from build123d import *

# Parameters (mm, degrees)
F1_DEPTH  = 35
F0_W      = 1.8
F0_H      = 39.6
F2_DEPTH  = 36
F0_W_2    = 30
F0_H_2    = 6.9
F3_DEPTH  = 1.8
F4_W      = 47.8
F4_H      = 28
F5_DEPTH  = 18
F4_W_2    = 50.8
F4_H_2    = 31.6
F6_DEPTH  = 1
F7_W      = 43.3
F7_H      = 39.6
F7_W_2    = 30
F7_H_2    = 48.3
F8_DEPTH  = 1.2
F0_W_3    = 6
F9_DEPTH  = 2
F10_R     = 1.6
F11_DEPTH = 2
F12_R     = 5.5
F13_DEPTH = 5
F10_R_2   = 4.5
F14_DEPTH = 2


with BuildPart() as f1:
    # F0 (on Top) → F1 (new body)
    with BuildSketch(Plane.XY):
        Polygon((-38.45, 21.6), (-38.45, 19.8), (-36.65, 19.8), (6.65, 19.8), (8.45, 19.8), (8.45, 21.6), (6.65, 21.6), align=None)
        Polygon((8.45, 21.6), (8.45, 19.8), (32.45, 19.8), (38.45, 19.8), (38.45, 21.6), align=None)
        Polygon((-36.65, -19.8), (-38.45, -19.8), (-38.45, -23.7), (40.25, -23.7), (40.25, 21.6), (38.45, 21.6), (38.45, 19.8), (38.45, -19.8), (32.45, -19.8), (12.45, -19.8), (12.45, -22.5), (-7.55, -22.5), (-7.55, -19.8), align=None)
    extrude(amount=F1_DEPTH)

    # F0 (on Top) → F2 (join)
    with BuildSketch(Plane.XY):
        with Locations((-37.55, 0)):
            Rectangle(F0_W, F0_H)
        Polygon((-38.45, 21.6), (-38.45, 19.8), (-36.65, 19.8), (6.65, 19.8), (8.45, 19.8), (8.45, 21.6), (6.65, 21.6), align=None)
        Polygon((6.65, 30.3), (6.65, 21.6), (8.45, 21.6), (8.45, 28.5), (38.45, 28.5), (38.45, 21.6), (40.25, 21.6), (40.25, 30.3), align=None)
        Polygon((-36.65, -19.8), (-38.45, -19.8), (-38.45, -23.7), (40.25, -23.7), (40.25, 21.6), (38.45, 21.6), (38.45, 19.8), (38.45, -19.8), (32.45, -19.8), (12.45, -19.8), (12.45, -22.5), (-7.55, -22.5), (-7.55, -19.8), align=None)
        Polygon((8.45, -19.8), (6.65, -19.8), (-7.55, -19.8), (-7.55, -22.5), (12.45, -22.5), (12.45, -19.8), align=None)
        with Locations((7.55, 0)):
            Rectangle(F0_W, F0_H)
    extrude(amount=-F2_DEPTH)

    # F0 (on Top) → F3 (join)
    with BuildSketch(Plane.XY):
        with Locations((23.45, 25.05)):
            Rectangle(F0_W_2, F0_H_2)
        Polygon((8.45, 21.6), (8.45, 19.8), (32.45, 19.8), (38.45, 19.8), (38.45, 21.6), align=None)
    extrude(amount=-F3_DEPTH)

    # F4 (on face) → F5 (cut)
    with BuildSketch(Plane.YZ.offset(40.25)):
        with Locations((3.3, -18)):
            Rectangle(F4_W, F4_H)
    extrude(amount=-F5_DEPTH, mode=Mode.SUBTRACT)

    # F4 (on face) → F6 (cut)
    with BuildSketch(Plane.YZ.offset(40.25)):
        with Locations((3.3, -18)):
            Rectangle(F4_W_2, F4_H_2)
        with Locations((3.3, -18)):
            Rectangle(F4_W, F4_H, mode=Mode.SUBTRACT)
    extrude(amount=-F6_DEPTH, mode=Mode.SUBTRACT)

    # F7 (on face) → F8 (join)
    with BuildSketch(Plane(origin=(0, 0, -36), x_dir=(1, 0, 0), z_dir=(0, 0, -1))):
        with Locations((-15, 0)):
            Rectangle(F7_W, F7_H)
        with Locations((23.45, -4.35)):
            Rectangle(F7_W_2, F7_H_2)
    extrude(amount=-F8_DEPTH)

    # F0 (on Top) → F9 (join)
    with BuildSketch(Plane.XY):
        with Locations((35.45, 0)):
            Rectangle(F0_W_3, F0_H)
    extrude(amount=-F9_DEPTH)

    # F10 (on face) → F11 (cut)
    with BuildSketch(Plane(origin=(0, 21.6, 0), x_dir=(-1, 0, 0), z_dir=(0, 1, 0))):
        with Locations((-35.25, 12.1)):
            Circle(F10_R)
    extrude(amount=-F11_DEPTH, mode=Mode.SUBTRACT)

    # F12 (on face) → F13 (cut)
    with BuildSketch(Plane(origin=(-38.45, 0, 0), x_dir=(0, -1, 0), z_dir=(-1, 0, 0))):
        with Locations((-3, -9)):
            Circle(F12_R)
        with Locations((16.8, -9)):
            Circle(F12_R)
        with Locations((6.9, -28.8)):
            Circle(F12_R)
    extrude(amount=-F13_DEPTH, mode=Mode.SUBTRACT)

    # F10 (on face) → F14 (cut)
    with BuildSketch(Plane(origin=(0, 21.6, 0), x_dir=(-1, 0, 0), z_dir=(0, 1, 0))):
        with Locations((-1.65, -14)):
            Circle(F10_R)
        with Locations((-1.65, -24)):
            Circle(F10_R)
        with Locations((31.45, -29)):
            Circle(F10_R_2)
    extrude(amount=-F14_DEPTH, mode=Mode.SUBTRACT)


solid = f1.part
The model under review builds one solid part; all positions refer to its coordinate system, in mm. A direction names the side the tool comes from. Round coordinates to 2 decimals unless told otherwise and drop trailing zeros. Write each loop counter-clockwise with the first axis right and the second up, starting at its lowest first coordinate (ties: lowest second). Pieces come first, ordered by that corner, then holes. Notation, with made-up numbers: M 16,67 L 27,67 A18 cw 27,82 Z; hole C 77.5,6 d11. An arc over 180 degrees is marked long. Use a Markdown table: item, result. Add a question column.
Q1. The part is to be moulded in two halves that separate along X. For faces 4 (the face through (39, -7, -4)), 5 (the face through (1.858, 20.713, -12.414)), say which applies: pulls with the +X half, pulls with the -X half, needs draft (parallel to the pull), parting line crosses it, or undercut.
Q2. We need section C-C, the plane x = 20.5. State the section outline as (y, z) points, plus the area to 3 significant figures.
Q3. We need section D-D, the plane y = 23. State the section outline as (x, z) points, plus the area to 3 significant figures.
Q4. Insertion check: pin 1 (12 mm diameter, centred on y = -2.5, z = 10.5, fed in from -X); pin 2 (4 mm diameter, centred on x = 1.65, z = -24, fed in from +Y); pin 3 (2 mm diameter, centred on x = -8, y = 15, fed in from +Z). Each pin has a flat end and moves straight along its axis. Give the tip position at first contact, or say it passes through.
Q5. Machinability: for faces 1 (the face through (-33.45, -21, -9)), 2 (the face through (32.45, 0, -1)), 3 (the face through (38.45, 8, -33)), which of the approach directions +Z, -Z, +X, -X, +Y, -Y give a long, thin tool a straight path to every point of the face, cutting with its end or side? Answer none if there is none.
Q6. To check wall thickness, follow line 1 (Z direction, x = 35.25, y = 20.55); line 2 (Y direction, x = -23.5, z = -1); line 3 (X direction, y = 3, z = -22.5). State the ranges of each line that lie inside material, in increasing order.
Q7. We need section B-B, the plane x = -31.45. State the section outline as (y, z) points.
Findings below:
| question | item | result |
|---|---|---|
| 1 | face 4 | needs draft |
| 1 | face 5 | undercut |
| 2 | outline | M -23.7,-36 L 30.3,-36 L 30.3,0 L 21.6,0 L 21.6,35 L 19.8,35 L 19.8,-1.8 L 28.5,-1.8 L 28.5,-34.8 L -19.8,-34.8 L -19.8,35 L -23.7,35 Z |
| 2 | area | 478 mm² |
| 3 | outline | M 6.65,-36 L 40.25,-36 L 40.25,-33.8 L 39.25,-33.8 L 39.25,-32 L 38.45,-32 L 38.45,-34.8 L 8.45,-34.8 L 8.45,-1.8 L 38.45,-1.8 L 38.45,-4 L 39.25,-4 L 39.25,-2.2 L 40.25,-2.2 L 40.25,0 L 6.65,0 Z |
| 3 | area | 166 mm² |
| 4 | pin 1 | stops at x = 38.45 |
| 4 | pin 2 | stops at y = 21.6 |
| 4 | pin 3 | stops at z = -34.8 |
| 5 | face 1 | -X |
| 5 | face 2 | +Z |
| 5 | face 3 | none |
| 6 | line 1 | z = -36 to -34.8, -1.8 to 10.5, 13.7 to 35 |
| 6 | line 2 | y = -23.7 to -19.8, 19.8 to 21.6 |
| 6 | line 3 | x = -38.45 to -36.65, 6.65 to 8.45 |
| 7 | outline | M -23.7,-36 L 21.6,-36 L 21.6,-33.5 L 19.8,-33.5 L 19.8,-34.8 L -19.8,-34.8 L -19.8,35 L -23.7,35 Z; M 19.8,-24.5 L 21.6,-24.5 L 21.6,35 L 19.8,35 Z |
